Work out the finished part from the listing and answer in its coordinate system (mm). Face numbers are marked on the shaded views. A direction names the side the tool comes from. Coordinates: 2 decimals unless noted, no trailing zeros. Order: outer loops, then holes, each group sorted by start corner. A loop starts at its lowest first (then second) coordinate and runs counter-clockwise, first axis right, second up. Notation, with made-up numbers: (-36.75, 87.5) -> (18.25, 87.5) arc R17 cw to (18.25, 99.5) -> close; hole circle Ø9 at (-12.75, 83). An arc over 180 degrees is marked (long way). Answer as CSV lines item,"result". Start each with the question number.
Item 1: Section D-D (z = 3) is taken. Write down the section's boundary in (x, y), then the cut area to 3 significant figures.
Item 2: Straight lines are drawn through the part: L1, parallel to Y at x = 0, z = 0.45; L2, parallel to X at y = 5, z = 1.25; L3, parallel to Y at x = 0, z = 1.15. For each, find the intervals that lie inside material, in ascending order.
Item 3: Each of these flat-tipped pins is pushed along its axis until it touches: pin 1 Ø1.1 at (y, z) = (22, -1) entering from +X; pin 2 Ø13 at (x, y) = (-3, -2.5) entering from +Z; pin 3 Ø1.1 at (x, z) = (-23.5, -1) entering from +Y; pin 4 Ø1.5 at (x, y) = (-17.5, -9.5) entering from +Z. Where does it stop, or does it pass through?
Item 4: Section A-A (y = 0) is taken. Write down the section's boundary in (x, z), then the cut area to 3 significant figures.
Item 5: Section C-C (x = 17.5) is taken. Write down the section's boundary in (y, z).
Item 6: Section B-B (x = 0) is taken. Write down the section's boundary in (y, z), then the cut area to 3 significant figures.
Item 7: Which of the six approach directions +Z, -Z, +X, -X, +Y, -Y give full straight-line access (tool end or side, diameter ignored) to the marked faces 1, 2, 3, 4 and 5?
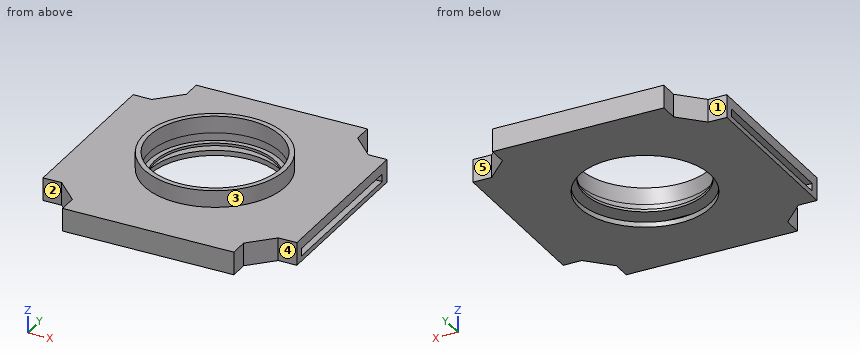
Autodesk Inventor part; units mm, degrees
ref_plane "YZ Plane" through (0, 0, 0) normal (1, 0, 0) x (0, 1, 0)
ref_plane "XZ Plane" through (0, 0, 0) normal (0, 1, 0) x (-1, 0, 0)
ref_plane "XY Plane" through (0, 0, 0) normal (0, 0, 1) x (1, 0, 0)
sketch "Sketch1" plane through (0, 0, 0) normal (0, 0, 1) x (1, 0, 0)
  line L0 (-34.8609, 0) -> (34.8609, 0) construction
  line L1 (0, -34.8609) -> (0, 34.8609) construction
  line L2 (0, 0) -> (13.4339, 13.4339) construction
  line L3 (0, 0) -> (18.9985, 0) construction
  line L4 (0, 24.9006) -> (16.8, 24.9006)
  line L5 (16.8, 24.9006) -> (16.8, 21.2406)
  line L6 (16.8, 21.2406) -> (19.0203, 19.0203)
  line L7 (24.9006, 0) -> (24.9006, 16.8)
  line L8 (24.9006, 16.8) -> (21.2406, 16.8)
  line L9 (21.2406, 16.8) -> (19.0203, 19.0203)
  line L10 (0, 0) -> (-13.4339, 13.4339) construction
  line L11 (0, 0) -> (-18.9985, 0) construction
  line L12 (0, 24.9006) -> (-16.8, 24.9006)
  line L13 (-16.8, 24.9006) -> (-16.8, 21.2406)
  line L14 (-16.8, 21.2406) -> (-19.0203, 19.0203)
  line L15 (-24.9006, 0) -> (-24.9006, 16.8)
  line L16 (-24.9006, 16.8) -> (-21.2406, 16.8)
  line L17 (-21.2406, 16.8) -> (-19.0203, 19.0203)
  line L18 (0, 0) -> (13.4339, -13.4339) construction
  line L19 (0, -24.9006) -> (16.8, -24.9006)
  line L20 (16.8, -24.9006) -> (16.8, -21.2406)
  line L21 (16.8, -21.2406) -> (19.0203, -19.0203)
  line L22 (24.9006, 0) -> (24.9006, -16.8)
  line L23 (24.9006, -16.8) -> (21.2406, -16.8)
  line L24 (21.2406, -16.8) -> (19.0203, -19.0203)
  line L25 (0, 0) -> (-13.4339, -13.4339) construction
  line L26 (0, -24.9006) -> (-16.8, -24.9006)
  line L27 (-16.8, -24.9006) -> (-16.8, -21.2406)
  line L28 (-16.8, -21.2406) -> (-19.0203, -19.0203)
  line L29 (-24.9006, 0) -> (-24.9006, -16.8)
  line L30 (-24.9006, -16.8) -> (-21.2406, -16.8)
  line L31 (-21.2406, -16.8) -> (-19.0203, -19.0203)
  dimension "d0" = 45
  dimension "d1" = 3.14
  dimension "d2" = 3.66
  dimension "d3" = 16.8
extrude "Extrusion1" add sketch "Sketch1" along normal blind 2 and the other way blind 2.5
hole "Hole1" at (0, 0, 0) direction (0, 0, 1) diameter 25.7 end through all both
sketch "Skizze3" plane through (24.9006, -16.8, 2) normal (1, 0, 0) x (0, 0, -1)
  line L0 (0, 33.6) -> (4.5, 33.6)
  line L1 (4.5, -4.4406) -> (4.5, 0)
  line L2 (2, 33.6) -> (4.5, 33.6) construction
  line L3 (2.7, 33.6) -> (2.7, 0) construction
  line L4 (2, 2.8) -> (2, 36.4349) construction
  line L5 (4.5, 33.6) -> (4.5, 0) construction
  line L6 (0, 0) -> (4.5, 0)
  line L7 (2, 31.8) -> (3.5, 31.8)
  line L8 (3.5, 31.8) -> (3.5, 1.8)
  line L9 (3.5, 1.8) -> (2, 1.8)
  line L10 (2, 1.8) -> (2, 31.8)
  point P0 (2, 16.8)
  point P1 (3.5, 16.8)
  point P2 (2.7, 16.8)
  point P3 (2, 16.8)
  point P4 (4.5, 16.8)
  dimension "d25" = 30
  dimension "d26" = 1.5
  dimension "d51" = 1
extrude "Extrusion3" cut sketch "Skizze3" against normal up to surface (49.8013 mm away)
sketch "Skizze4" plane through (24.9006, -15, 0) normal (0, 0, -1) x (-1, 0, 0)
  circle A0 centre (24.9006, 15) radius 11.85
  circle A1 centre (24.9006, 15) radius 12.85
  dimension "d33" = 23.7
  dimension "d34" = 1
extrude "Extrusion4" add sketch "Skizze4" against normal blind 0.5
sketch "Sketch7" plane through (0, 0, 2) normal (0, 0, 1) x (1, 0, 0)
  circle A0 centre (0, 0) radius 12.85 construction
  circle A1 centre (0, 0) radius 12.85
  circle A2 centre (0, 0) radius 13.85
  dimension "d52" = 25.7
  dimension "d53" = 1
extrude "Extrusion7" add sketch "Sketch7" along normal blind 3.3
equation "\"Lens_diameter\" = 25"
properties part number "polarbox_20_Lens_holder 1st design"
Checked values:
1,outline,"circle Ø27.7 at (0, 0); hole circle Ø25.7 at (0, 0)"
1,area,"83.9 mm^2"
2,L1,"y = -24.9 to -11.85, 11.85 to 24.9"
2,L2,"x = -24.9 to -11.84, 11.84 to 24.9"
2,L3,"y = -24.9 to -12.85, 12.85 to 24.9"
3,pin 1,"stops at x = 16.8"
3,pin 2,"passes through"
3,pin 3,"stops at y = 16.8"
3,pin 4,"stops at z = 2"
4,outline,"(-24.9, -2.5) -> (-12.85, -2.5) -> (-12.85, -1.5) -> (-24.9, -1.5) -> close; (-24.9, 0) -> (-11.85, 0) -> (-11.85, 0.5) -> (-12.85, 0.5) -> (-12.85, 5.3) -> (-13.85, 5.3) -> (-13.85, 2) -> (-24.9, 2) -> close; (11.85, 0) -> (24.9, 0) -> (24.9, 2) -> (13.85, 2) -> (13.85, 5.3) -> (12.85, 5.3) -> (12.85, 0.5) -> (11.85, 0.5) -> close; (12.85, -2.5) -> (24.9, -2.5) -> (24.9, -1.5) -> (12.85, -1.5) -> close"
4,area,"79.9 mm^2"
5,outline,"(-20.54, -2.5) -> (20.54, -2.5) -> (20.54, 2) -> (-20.54, 2) -> close; hole (-15, -1.5) -> (15, -1.5) -> (15, 0) -> (-15, 0) -> close"
6,outline,"(-24.9, -2.5) -> (-12.85, -2.5) -> (-12.85, -1.5) -> (-15, -1.5) -> (-15, 0) -> (-11.85, 0) -> (-11.85, 0.5) -> (-12.85, 0.5) -> (-12.85, 5.3) -> (-13.85, 5.3) -> (-13.85, 2) -> (-24.9, 2) -> close; (11.85, 0) -> (15, 0) -> (15, -1.5) -> (12.85, -1.5) -> (12.85, -2.5) -> (24.9, -2.5) -> (24.9, 2) -> (13.85, 2) -> (13.85, 5.3) -> (12.85, 5.3) -> (12.85, 0.5) -> (11.85, 0.5) -> close"
6,area,"110 mm^2"
7,face 1,"+Z, -Z, -X, +Y"
7,face 2,"+Z, -Z, -X, -Y"
7,face 3,"+Z"
7,face 4,"+Z, -Z, +X, -Y"
7,face 5,"+Z, -Z, +X, +Y"
